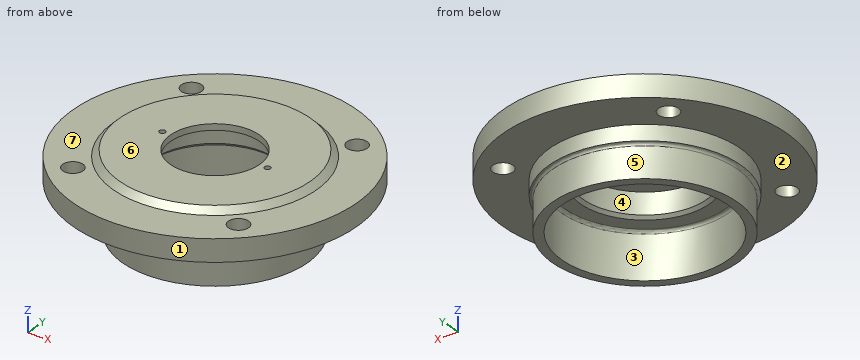
```python
from build123d import *

# Parameters (mm, degrees)
M6_CLEARANCE_HOLE1_D = 6.6
CIRPATTERN1_COUNT    = 4
CUT_EXTRUDE1_REACH   = 71.764
SKETCH5_R            = 1


with BuildPart() as part:
    # Sketch1 → Revolve1 (revolve)
    with BuildSketch(Plane(origin=(0, 0, 0), x_dir=(0, 0, -1), z_dir=(1, 0, 0)), mode=Mode.PRIVATE) as revolve1_sk:
        with BuildLine():
            Line((0, 14.5), (0, 31))
            Line((0, 31), (2, 33))
            Line((2, 33), (2, 46))
            Line((2, 46), (9.2, 46))
            Line((9.2, 46), (9.2, 31))
            Line((9.2, 31), (14.2, 31))
            ThreePointArc((14.2, 31), (14.492893219, 30.292893219), (15.2, 30))
            Line((15.2, 30), (25.2, 30))
            Line((25.2, 30), (25.2, 27))
            Line((25.2, 27), (11, 27))
            ThreePointArc((11, 27), (10.292893219, 26.707106781), (10, 26))
            Line((10, 26), (10, 21))
            Line((10, 21), (9, 20))
            Line((9, 20), (2, 20))
            Line((2, 20), (2, 14.5))
            Line((2, 14.5), (0, 14.5))
        make_face()
    revolve(revolve1_sk.sketch.rotate(Axis((0, 0, 0), (0, 0, -1)), 180), axis=Axis((0, 0, 0), (0, 0, -1)))

    # M6 Clearance Hole1 (through all)
    with Locations(Plane.XY.offset(-2)):
        with Locations((27.223611076, 27.223611076)):
            m6_clearance_hole1 = Hole(M6_CLEARANCE_HOLE1_D / 2)

    # CirPattern1: M6 Clearance Hole1 ×4 about axis
    cirpattern1_axis = Axis((0, 0, 0), (0, 0, 1))
    for i in range(1, CIRPATTERN1_COUNT):
        add(m6_clearance_hole1.rotate(cirpattern1_axis, i * 360 / CIRPATTERN1_COUNT), mode=Mode.SUBTRACT)

    # Sketch5 → Cut-Extrude1 (cut, up to next)
    with BuildSketch(Plane.XY, mode=Mode.PRIVATE) as cut_extrude1_sk1:
        with Locations((17.27, 0)):
            Circle(SKETCH5_R)
    cut_extrude1_tool1 = extrude(cut_extrude1_sk1.sketch, amount=-CUT_EXTRUDE1_REACH, mode=Mode.PRIVATE) & part.part
    # Sketch5 → Cut-Extrude1 (cut, up to next)
    with BuildSketch(Plane.XY, mode=Mode.PRIVATE) as cut_extrude1_sk2:
        with Locations(Location((-17.27, 0, 0), (0, 0, 270))):
            Circle(SKETCH5_R)
    cut_extrude1_tool2 = extrude(cut_extrude1_sk2.sketch, amount=-CUT_EXTRUDE1_REACH, mode=Mode.PRIVATE) & part.part
    add(cut_extrude1_tool1.solids().sort_by_distance((17.27, 0, 0))[0], mode=Mode.SUBTRACT)
    add(cut_extrude1_tool2.solids().sort_by_distance((-17.27, 0, 0))[0], mode=Mode.SUBTRACT)


solid = part.part
```
CAD build for the part. Positions are in the model's coordinates, mm. Face numbers are marked on the shaded views. A direction names the side the tool comes from. Coordinates: 2 decimals unless noted, no trailing zeros. Order: outer loops, then holes, each group sorted by start corner. A loop starts at its lowest first (then second) coordinate and runs counter-clockwise, first axis right, second up. Notation, with made-up numbers: M 62.5,58 L 88.5,58 A16 cw 88.5,62 Z; hole C -16,74.5 d7. An arc over 180 degrees is marked long. Answer as CSV lines item,"result".
1) Drill centre lines: L1, parallel to X at y = 0, z = -21.75; L2, parallel to Z at x = -17, y = 5.5; L3, parallel to Z at x = -28, y = -32. Where is each one in solid material? Low to high. Write a range as from..to.
Verdict:
L1,"-30..-27, 27..30"
L2,"-2..0"
L3,"-9.2..-2"
2) 3-axis set-ups, long thin cutter, end or side, ignore diameter. For the marked faces 5, 6 and 7: which of +Z, -Z, +X, -X, +Y, -Y reach the whole face in a straight line?
Verdict:
face 5,"-Z"
face 6,"+Z, +X, -X, +Y, -Y"
face 7,"+Z"
3) Cut at C-C (z = -6.75). List the corners of the cut face in (x, y).
Verdict:
outline,"C 0,0 d92; hole C -27.22,-27.22 d6.6; hole C -27.22,27.22 d6.6; hole C 0,0 d40; hole C 27.22,-27.22 d6.6; hole C 27.22,27.22 d6.6"
4) Cut at B-B (z = -16.75). List the corners of the cut face in (x, y), then the cut area to 3 significant figures.
Verdict:
outline,"C 0,0 d60; hole C 0,0 d54"
area,"537 mm2"
5) Mould opens along X. For the marked faces 1, 2, 3 and 4 say: released by +X, released by -X, zero draft, split by the parting line, or undercut.
Verdict:
face 1,"split by the parting line"
face 2,"zero draft"
face 3,"undercut"
face 4,"undercut"
6) Flat gauge pins, fed straight in: P1, Ø6, axis at y = 25.5, z = -15.5, coming from the -X side; P2, Ø4, axis at x = 27.5, y = 33.5, coming from the +Z side; P3, Ø3, axis at x = -17.27, y = 0, coming from the -Z side. Where does each tip first touch, or does it go through?
Verdict:
P1,"x = -21.01"
P2,"z = -2"
P3,"z = -2"
